Study the drawing (mm; zero at the part's minimum x, y, z) and answer. Coordinates: 2 decimals unless noted, no trailing zeros. Order: outer loops, then holes, each group sorted by start corner. A loop starts at its lowest first (then second) coordinate and runs counter-clockwise, first axis right, second up. Notation, with made-up numbers: M 25.25,22 L 67.25,22 A30 ccw 67.25,50 Z; hole C -16.75,-28.5 d7. An arc over 180 degrees is marked long. Put each result on its own line as item: value.
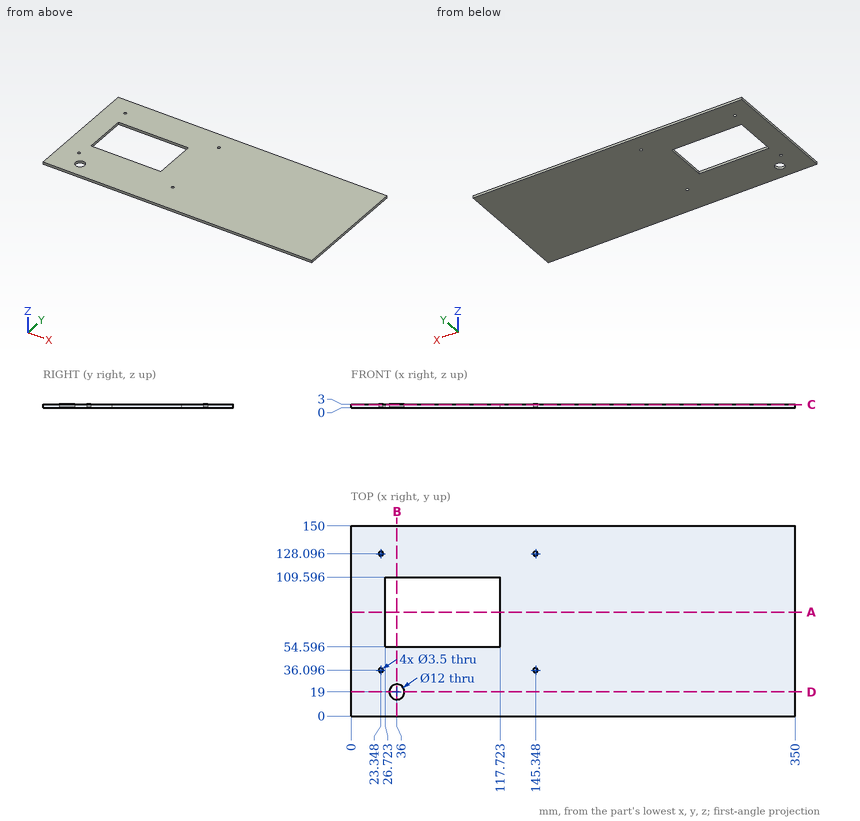
Q1. Find section B-B on x = 36. Write down the section's boundary in (y, z) (1 decimal).
Answers below:
outline: M 0,0 L 13,0 L 13,3 L 0,3 Z; M 25,0 L 54.6,0 L 54.6,3 L 25,3 Z; M 109.6,0 L 150,0 L 150,3 L 109.6,3 Z
Q2. Find section C-C on z = 2.45. Give the number of separate pieces and of enclosed holes in the cut face, plus the area to 3 significant figures.
Answers below:
separate pieces: 1
enclosed holes: 6
area: 47,300 mm^2
Q3. Find section A-A on y = 82. Write down the section's boundary in (x, z).
Answers below:
outline: M 0,0 L 26.72,0 L 26.72,3 L 0,3 Z; M 117.72,0 L 350,0 L 350,3 L 117.72,3 Z
Q4. Consider line 1 along X through (y, z) = (58, 1.35); line 2 along Y through (x, z) = (114.5, 1.6) (1 decimal); line 3 along X through (y, z) = (127, 1.15) (1 decimal). Determine where each line is inside the solid, lowest interval first.
Answers below:
line 1: x = 0 to 26.72, 117.72 to 350
line 2: y = 0 to 54.6, 109.6 to 150
line 3: x = 0 to 22, 24.7 to 144, 146.7 to 350
Q5. Find section D-D on y = 19. Write down the section's boundary in (x, z), plus the area to 3 significant figures.
Answers below:
outline: M 0,0 L 30,0 L 30,3 L 0,3 Z; M 42,0 L 350,0 L 350,3 L 42,3 Z
area: 1,010 mm^2
Q6. Given pin 1 (6 mm diameter, centred on x = 69.5, y = 23, fed in from -Z); pin 2 (2 mm diameter, centred on x = 145.35, y = 128.1, fed in from +Z) (1 decimal), each flat-ended and moving along its own axis, determine where each tip first touches the part or whether it passes through.
Answers below:
pin 1: stops at z = 0
pin 2: passes through
